Geometry check sheet. Reference: the model listing, model coordinates, mm. Give positions to 0.01 mm unless a question says otherwise; leave off trailing zeros. Loops run counter-clockwise (first coordinate to the right, second up) from the corner with the lowest first, then second, coordinate; pieces in that order, holes last.
1. Cross-section at C-C, the plane z = -156.75. Record the cut outline in (x, y) (3 decimals).
2. Go/stop test with flat-tipped pins: pin 1 Ø1 at (x, y) = (87, 0) entering from -Z; pin 2 Ø2 at (x, z) = (78.5, -162.5) entering from -Y. Record where each tip stops, or that it passes through.
3. Material ranges on L1, parallel to X at y = 1, z = -151.75; L2, parallel to Z at x = 88.5, y = 2.5; L3, parallel to Z at x = 89, y = -2.5, recorded low to high.
4. Release check for a two-part mould opening along Z. For faces 1 (the flat face through (104.563, -0.044, -155.708)), 2 (the flat face through (88, -3.175, -155)), 3 (the flat face through (99, 0, -165.1)) record: +Z half, -Z half, draft (parallel to the pull), parting line (faces both ways), or undercut.
5. Cross-section at B-B, the plane x = 83.5. Record the cut outline in (y, z) (1 decimal), plus the area to 3 significant figures.
from build123d import *

# Parameters (mm, degrees)
F1_DEPTH = 3.175


with BuildPart() as f1:
    # F0 (on Front) → F1 (new body, symmetric)
    with BuildSketch(Plane.XZ):
        with BuildLine():
            ThreePointArc((81.6381810245, -141.4014773719), (76.9896583964, -146.05), (75.2881810245, -152.4))
            Line((75.2881810245, -152.4), (86.4006810245, -152.4))
            ThreePointArc((86.4006810245, -152.4), (86.613365696, -151.60625), (87.1944310245, -151.0251846715))
            Line((87.1944310245, -151.0251846715), (81.6381810245, -141.4014773719))
        make_face()
        with BuildLine():
            ThreePointArc((76.9896583964, -158.75), (81.6381810245, -163.3985226281), (87.9881810245, -165.1))
            ThreePointArc((87.9881810245, -165.1), (96.9684371456, -161.3802561211), (100.6881810245, -152.4))
            ThreePointArc((100.6881810245, -152.4), (100.2554390184, -149.1129981272), (98.9867036526, -146.05))
            ThreePointArc((98.9867036526, -146.05), (94.3381810245, -141.4014773719), (87.9881810245, -139.7))
            ThreePointArc((87.9881810245, -139.7), (84.7011791517, -140.1327420061), (81.6381810245, -141.4014773719))
            Line((81.6381810245, -141.4014773719), (87.1944310245, -151.0251846715))
            ThreePointArc((87.1944310245, -151.0251846715), (88.7819310245, -151.0251846715), (89.5756810245, -152.4))
            ThreePointArc((89.5756810245, -152.4), (87.9881810245, -153.9875), (86.4006810245, -152.4))
            Line((86.4006810245, -152.4), (75.2881810245, -152.4))
            ThreePointArc((75.2881810245, -152.4), (75.7209230306, -155.6870018728), (76.9896583964, -158.75))
        make_face()
        with BuildLine():
            Line((87.9881810245, -139.7), (80.6558326058, -139.7))
            Line((80.6558326058, -139.7), (81.6381810245, -141.4014773719))
            ThreePointArc((81.6381810245, -141.4014773719), (84.7011791517, -140.1327420061), (87.9881810245, -139.7))
        make_face()
        with BuildLine():
            Line((80.6558326058, -139.7), (65.9911357684, -139.7))
            Line((65.9911357684, -139.7), (73.3234841871, -152.4))
            Line((73.3234841871, -152.4), (75.2881810245, -152.4))
            ThreePointArc((75.2881810245, -152.4), (76.9896583964, -146.05), (81.6381810245, -141.4014773719))
            Line((81.6381810245, -141.4014773719), (80.6558326058, -139.7))
        make_face()
        with BuildLine():
            Line((75.2881810245, -152.4), (73.3234841871, -152.4))
            Line((73.3234841871, -152.4), (76.9896583964, -158.75))
            ThreePointArc((76.9896583964, -158.75), (75.7209230306, -155.6870018728), (75.2881810245, -152.4))
        make_face()
        with BuildLine():
            ThreePointArc((100.6881810245, -152.4), (96.9684371456, -161.3802561211), (87.9881810245, -165.1))
            Line((87.9881810245, -165.1), (109.9852262806, -165.1))
            Line((109.9852262806, -165.1), (98.9867036526, -146.05))
            ThreePointArc((98.9867036526, -146.05), (100.2554390184, -149.1129981272), (100.6881810245, -152.4))
        make_face()
    extrude(amount=F1_DEPTH, both=True)


solid = f1.part
Result:
1. outline: (75.835, -3.175) - (105.164, -3.175) - (105.164, 3.175) - (75.835, 3.175) - close
2. pin 1: stops at z = -165.09
2. pin 2: passes through
3. L1: x = 72.95 to 86.54, 89.44 to 102.28
3. L2: z = -165.1 to -153.9, -150.9 to -139.71
3. L3: z = -165.1 to -153.62, -151.18 to -139.74
4. face 1: +Z half
4. face 2: draft
4. face 3: -Z half
5. outline: (-3.2, -164.3) - (3.2, -164.3) - (3.2, -139.7) - (-3.2, -139.7) - close
5. area: 156 mm2
